Read the model definition and answer for the solid it produces. Units are mm, in the model's axes. Face numbers are marked on the shaded views. A direction names the side the tool comes from. Coordinates: 2 decimals unless noted, no trailing zeros. Loops run counter-clockwise (first coordinate to the right, second up) from the corner with the lowest first, then second, coordinate; pieces in that order, holes last. Notation, with made-up numbers: (-17, 21) -> (14, 21) arc R10 cw to (14, 30) -> close; hole circle Ø4 at (-6.5, 14.25). An arc over 180 degrees is marked (long way). One line per question, with ' | ' between items. Start each with the question number.
```python
from build123d import *

# Parameters (mm, degrees)
F0_R     = 4.5
F0_R_2   = 2.4
F1_DEPTH = 2.5
F2_DEPTH = 5
F0_W     = 2
F0_H     = 100
F3_DEPTH = 2
F4_W     = 40.8
F4_H     = 5
F5_DEPTH = 15
F6_W     = 40.8
F6_H     = 10
F7_DEPTH = 5
F8_R     = 4.99999
F9_R     = 2


# Not quite as in the source:
# - a fillet or chamfer is up to 0.001 mm smaller than in the source, because OpenCascade refuses the exact size


with BuildPart() as f1:
    # F0 (on Top) → F1 (new body)
    with BuildSketch(Plane.XY):
        Circle(F0_R)
        Circle(F0_R_2, mode=Mode.SUBTRACT)
    extrude(amount=F1_DEPTH)

    # F0 (on Top) → F2 (join)
    with BuildSketch(Plane.XY):
        Polygon((-10, -50), (10, -50), (10, 50), (0, 50), (-10, 50), align=None)
        Circle(F0_R, mode=Mode.SUBTRACT)
        Polygon((0, 50), (10, 50), (12, 50), (20.4, 50), (20.4, 60), (-20.4, 60), (-20.4, 50), (-12, 50), (-10, 50), align=None)
    extrude(amount=F2_DEPTH)

    # F0 (on Top) → F3 (join)
    with BuildSketch(Plane.XY):
        with Locations((-11, 0)):
            Rectangle(F0_W, F0_H)
        with Locations((11, 0)):
            Rectangle(F0_W, F0_H)
    extrude(amount=F3_DEPTH)

    # F4 (on face) → F5 (join)
    with BuildSketch(Plane.XY.offset(5)):
        with Locations((0, 57.5)):
            Rectangle(F4_W, F4_H)
    extrude(amount=F5_DEPTH)

    # F6 (on face) → F7 (join)
    with BuildSketch(Plane.XY.offset(20)):
        with Locations((0, 55)):
            Rectangle(F6_W, F6_H)
    extrude(amount=F7_DEPTH)

    # F8 (radius 5 in the source; OpenCascade refuses exactly that, so slightly less here)
    f8_edges = [f1.edges().sort_by_distance(p)[0] for p in [
        (-20.4, 50, 22.5),
        (20.4, 50, 22.5),
        (0, 60, 25),
        (0, 60, 0),
    ]]
    fillet(f8_edges, radius=F8_R)

    # F9
    f9_edges = [f1.edges().sort_by_distance(p)[0] for p in [
        (-20.4, 55, 12.5),
        (20.4, 55, 12.5),
        (-12, -50, 1),
        (12, -50, 1),
        (-10, -50, 3.5),
        (10, -50, 3.5),
        (-20.4, 50, 2.5),
        (20.4, 50, 2.5),
    ]]
    fillet(f9_edges, radius=F9_R)


solid = f1.part
```
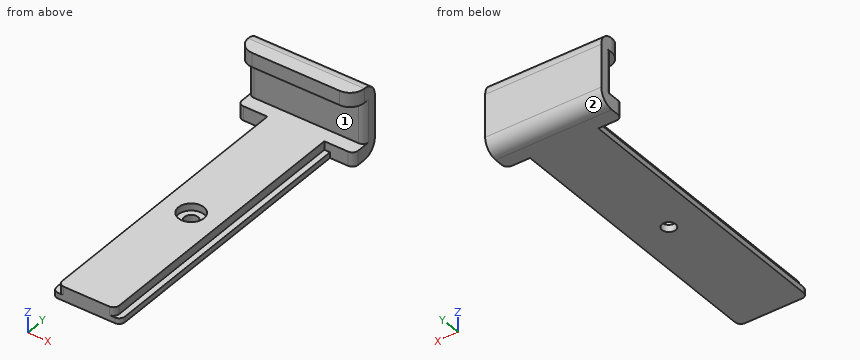
(1) Section D-D on z = 13.5 is taken. Write down the section's boundary in (x, y).
(2) Each of these flat-tipped pins is pushed along its axis until it touches: pin 1 Ø2.5 at (x, z) = (16, 2) entering from -Y; pin 2 Ø3 at (x, y) = (10.5, 3) entering from +Z; pin 3 Ø1.5 at (y, z) = (19, 4) entering from +X. Where does it stop, or does it pass through?
(3) A tool of negligible diameter and unlimited length cuts with its end or side. For the marked faces 1 and 2, from which of +Z, -Z, +X, -X, +Y, -Y can it reach the whole face along a straight path? Write none if from no direction.
(4) Section C-C on y = -19 is taken. Write down the section's boundary in (x, z), plus the area to 3 significant figures.
(5) Section A-A on x = 0 is taken. Write down the section's boundary in (y, z), plus the area to 3 significant figures.
(6) Find the intervals of material crossed by probe 1 along Z at (x, y) = (5.5, 51); probe 2 along Z at (x, y) = (0, 49.5); probe 3 along Y at (x, z) = (-10, 12.5), in increasing order. Write a range as from..to.
(7) Section B-B on y = 0 is taken. Write down the section's boundary in (x, z).
Working result:
1) outline: (-20.4, 57) arc R2 ccw to (-18.4, 55) -> (18.4, 55) arc R2 ccw to (20.4, 57) -> (20.4, 60) -> (-20.4, 60) -> close
2) pin 1: stops at y = 50 | pin 2: stops at z = 5 | pin 3: stops at x = 10
3) face 1: +X, -X, -Y | face 2: -Z, +X, -X, +Y
4) outline: (-12, 0) -> (12, 0) -> (12, 2) -> (10, 2) -> (10, 5) -> (-10, 5) -> (-10, 2) -> (-12, 2) -> close | area: 108 mm2
5) outline: (-50, 0) -> (-2.4, 0) -> (-2.4, 2.5) -> (-4.5, 2.5) -> (-4.5, 5) -> (-50, 5) -> close; (2.4, 0) -> (55, 0) arc R5 ccw to (60, 5) -> (60, 20) arc R5 ccw to (55, 25) -> (50, 25) -> (50, 20) -> (55, 20) -> (55, 5) -> (4.5, 5) -> (4.5, 2.5) -> (2.4, 2.5) -> close | area: 630 mm2
6) probe 1: z = 0..5, 20..25 | probe 2: z = 0..5 | probe 3: y = 55..60
7) outline: (-12, 0) -> (-2.4, 0) -> (-2.4, 2.5) -> (-4.5, 2.5) -> (-4.5, 5) -> (-10, 5) -> (-10, 2) -> (-12, 2) -> close; (2.4, 0) -> (12, 0) -> (12, 2) -> (10, 2) -> (10, 5) -> (4.5, 5) -> (4.5, 2.5) -> (2.4, 2.5) -> close
